Autodesk Inventor part; units mm, degrees
ref_plane "YZ Plane" through (0, 0, 0) normal (1, 0, 0) x (0, 1, 0)
ref_plane "XZ Plane" through (0, 0, 0) normal (0, 1, 0) x (-1, 0, 0)
ref_plane "XY Plane" through (0, 0, 0) normal (0, 0, 1) x (1, 0, 0)
sketch "Эскиз1" plane through (0, 0, 0) normal (0, 0, 1) x (1, 0, 0)
  circle A0 centre (0, 0) radius 30
  dimension "d0" = 60
extrude "Выдавливание1" add sketch "Эскиз1" along normal blind 2
sketch "Эскиз2" plane through (0, 0, 2) normal (0, 0, 1) x (1, 0, 0)
  circle A0 centre (0, 0) radius 20
  dimension "d3" = 40
extrude "Выдавливание2" add sketch "Эскиз2" along normal blind 2
sketch "Эскиз3" plane through (0, 0, 4) normal (0, 0, 1) x (1, 0, 0)
  circle A0 centre (7.2251, 12.5143) radius 1
  line L0 (-42, 0) -> (42, 0)
  line L1 (0, -42) -> (0, 42)
  line L2 (0, 0) -> (7.2251, 12.5143)
  dimension "d6" = 2
  dimension "d10" = 30
extrude "Выдавливание3" cut sketch "Эскиз3" against normal through all
properties part number "Для регулировки 4" material "Сталь, высокопрочная, низколегированная"
Build history of the part. All positions in model axes, mm. A direction names the side the tool comes from. Coordinates: 2 decimals unless noted, no trailing zeros. Order: outer loops, then holes, each group sorted by start corner. A loop starts at its lowest first (then second) coordinate and runs counter-clockwise, first axis right, second up.
Item 1: Drill centre lines: L1, parallel to Z at x = -12, y = 18.5; L2, parallel to Y at x = 0, z = 3.35; L3, parallel to X at y = 12, z = 3.15. Where is each one in solid material? Low to high.
Filled in:
L1: z = 0 to 2
L2: y = -20 to 20
L3: x = -16 to 6.37, 8.08 to 16
Item 2: Tool access for faces 4 (the cylindrical face through (-4.336, 19.524, 2.986)), 5 (the flat face through (0, 0, 4)): list every direction of +Z, -Z, +X, -X, +Y, -Y with a clear straight run to the whole face (end or side of a thin tool).
Filled in:
face 4: +Z
face 5: +Z, +X, -X, +Y, -Y
Item 3: Drop flat-ended pins along their axis: pin 1 Ø5 at (x, y) = (2, 4.5) entering from -Z; pin 2 Ø2 at (y, z) = (4.5, 2.5) entering from +X; pin 3 Ø1.6 at (x, y) = (7.23, 12.51) entering from +Z (3 decimals). Give the stop position or say it passes through.
Filled in:
pin 1: stops at z = 0
pin 2: stops at x = 29.78
pin 3: passes through
Item 4: Saw through at A-A on y = 0. List the corners of the cut face in (x, z), then the cut area to 3 significant figures.
Filled in:
outline: (-30, 0) - (30, 0) - (30, 2) - (20, 2) - (20, 4) - (-20, 4) - (-20, 2) - (-30, 2) - close
area: 200 mm2
Item 5: Mould opens along Y. For faces 1 (the flat face through (6, -20, 2)), 2 (the cylindrical face through (7.008, 11.538, 2.028)), 3 (the cylindrical face through (-29.97, -1.32, 0.99)) say: released by +Y, released by -Y, zero draft, split by the parting line, or undercut.
Filled in:
face 1: zero draft
face 2: undercut
face 3: split by the parting line
Item 6: Saw through at C-C on z = 3. List the corners of the cut face in (x, y).
Filled in:
outline: circle Ø40 at (0, 0); hole circle Ø2 at (7.23, 12.51)
